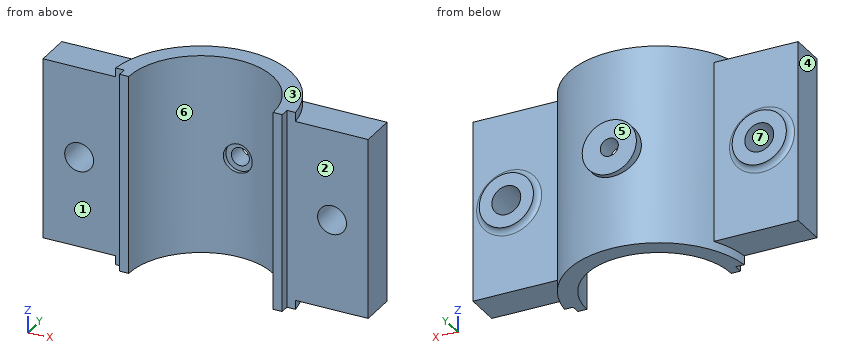
from build123d import *

# Parameters (mm, degrees)
BOSS_EXTRUDE1_DEPTH      = 55
SKETCH2_W                = 180
SKETCH2_H                = 20
BOSS_EXTRUDE2_DEPTH      = 50
SKETCH3_W                = 5
SKETCH3_H                = 5
CUT_EXTRUDE1_DEPTH       = 151.665191733
CUT_EXTRUDE2_DEPTH       = 151.665191733
CUT_EXTRUDE2_DEPTH_BACK  = 151.665191733
SKETCH5_R                = 15
BOSS_EXTRUDE3_DEPTH      = 3
BOSS_EXTRUDE4_REACH      = 120.042
BOSS_EXTRUDE4_END_RADIUS = 50
SKETCH6_R                = 15
HOLE1_D                  = 10
HOLE2_D                  = 16
FILLET1_R                = 3
SKETCH11_R               = 8
CUT_EXTRUDE3_DEPTH       = 42


with BuildPart() as part:
    # Sketch1 → Boss-Extrude1 (new, symmetric)
    with BuildSketch(Plane.XY):
        with BuildLine():
            Line((-50, 0), (50, 0))
            ThreePointArc((50, 0), (0, 50), (-50, 0))
        make_face()
    extrude(amount=BOSS_EXTRUDE1_DEPTH, both=True)

    # Sketch2 → Boss-Extrude2 (add, symmetric)
    with BuildSketch(Plane.XY):
        with Locations((0, 15)):
            Rectangle(SKETCH2_W, SKETCH2_H)
    extrude(amount=BOSS_EXTRUDE2_DEPTH, both=True)

    # Sketch3 → Cut-Extrude1 (cut, symmetric)
    with BuildSketch(Plane.XY.offset(55)):
        with Locations((47.5, 2.5)):
            Rectangle(SKETCH3_W, SKETCH3_H)
    cut_extrude1 = extrude(amount=CUT_EXTRUDE1_DEPTH, both=True, mode=Mode.SUBTRACT)

    # Mirror1: Cut-Extrude1 across plane
    add(cut_extrude1.mirror(Plane(origin=(0, 0, 0), x_dir=(0, 0, 1), z_dir=(1, 0, 0))), mode=Mode.SUBTRACT)

    # Sketch4 → Cut-Extrude2 (cut, two sides: drawn at the far end of the back side and taken through both)
    with BuildSketch(Plane.XY.offset(55).offset(-CUT_EXTRUDE2_DEPTH_BACK)):
        with BuildLine():
            Line((40, 0), (-40, 0))
            ThreePointArc((-40, 0), (0, 40), (40, 0))
        make_face()
    extrude(amount=CUT_EXTRUDE2_DEPTH + CUT_EXTRUDE2_DEPTH_BACK, mode=Mode.SUBTRACT)

    # Sketch5 → Boss-Extrude3 (add)
    with BuildSketch(Plane(origin=(0, 25, 0), x_dir=(1, 0, 0), z_dir=(0, 1, 0))):
        with Locations(Location((-70, 0, 0), (0, 0, 90))):
            Circle(SKETCH5_R)
    boss_extrude3 = extrude(amount=BOSS_EXTRUDE3_DEPTH)

    # Mirror2: Boss-Extrude3 across plane
    add(boss_extrude3.mirror(Plane(origin=(0, 0, 0), x_dir=(0, 0, 1), z_dir=(1, 0, 0))))

    # Boss-Extrude4: up to this cylinder (the profile starts outside it)
    boss_extrude4_end = Plane(origin=(0, 0, 0), z_dir=(0, 0, -1)) * Cylinder(BOSS_EXTRUDE4_END_RADIUS, 341.084, mode=Mode.PRIVATE)
    # Sketch6 → Boss-Extrude4 (add, up to the surface)
    with BuildSketch(Plane(origin=(0, 53, 0), x_dir=(1, 0, 0), z_dir=(0, 1, 0)), mode=Mode.PRIVATE) as boss_extrude4_sk1:
        with Locations(Location((0, 0, 0), (0, 0, 270))):
            Circle(SKETCH6_R)
    boss_extrude4_tool1 = extrude(boss_extrude4_sk1.sketch, amount=-BOSS_EXTRUDE4_REACH, mode=Mode.PRIVATE) - boss_extrude4_end
    add(boss_extrude4_tool1.solids().sort_by_distance((0, 53, 0))[0])

    # Hole1 (through all)
    with Locations(Plane(origin=(0, 53, 0), x_dir=(1, 0, 0), z_dir=(0, 1, 0))):
        with Locations((0, 0)):
            Hole(HOLE1_D / 2)

    # Hole2 (through all)
    with Locations(Plane(origin=(0, 28, 0), x_dir=(1, 0, 0), z_dir=(0, 1, 0))):
        with Locations((-70, 0), (70, 0)):
            Hole(HOLE2_D / 2)

    # Fillet1
    fillet1_edges = [part.edges().sort_by_distance(p)[0] for p in [
        (-70, 25, 15),
        (70, 25, 15),
    ]]
    fillet(fillet1_edges, radius=FILLET1_R - 0.0001)  # a hair under: the kernel refuses the full size

    # Sketch11 → Cut-Extrude3 (cut)
    with BuildSketch(Plane(origin=(0, 0, 0), x_dir=(1, 0, 0), z_dir=(0, 1, 0))):
        with Locations(Location((0, 0, 0), (0, 0, 90))):
            Circle(SKETCH11_R)
    extrude(amount=CUT_EXTRUDE3_DEPTH, mode=Mode.SUBTRACT)


solid = part.part
CAD build for the part. Positions are in the model's coordinates, mm. Face numbers are marked on the shaded views. A direction names the side the tool comes from. Round coordinates to 2 decimals unless told otherwise and drop trailing zeros. Loops run counter-clockwise (first coordinate to the right, second up) from the corner with the lowest first, then second, coordinate; pieces in that order, holes last. Notation, with made-up numbers: M 2.5,-15 L 21.5,-15 A20 cw 21.5,7 Z; hole C -18,48.5 d9. An arc over 180 degrees is marked long. One line per question, with ' | ' between items. Start each with the question number.
Item 1: Pin check, flat tips, straight feed: pin 1 Ø17.5 at (x, z) = (4, 3) entering from -Y; pin 2 Ø1 at (y, z) = (30, 15) entering from +X; pin 3 Ø9 at (x, z) = (77, 7) entering from +Y. Stop position of each tip, or through.
Item 2: Two-plate mould, pull along X, no slides. Class the marked faces 4, 5, 6 and 7: pulls with the +X half, pulls with the -X half, needs draft (parallel to the pull), parting line crosses it, or undercut.
Item 3: Cut at D-D, the plane x = -47.5. Write the cut outline in (y, z), plus the area to 3 significant figures.
Item 4: Cut at C-C, the plane z = -38.5. Write the cut outline in (x, y).
Item 5: Wall check: line 1 (Z direction, x = 0, y = 49); line 2 (Y direction, x = -69, z = 30.5); line 3 (Z direction, x = 56.5, y = 8). Give the ranges that are in metal, low to high.
Item 6: Cut at B-B, the plane y = 20. Write the cut outline in (x, z).
Item 7: Which spindle directions (+Z, -Z, +X, -X, +Y, -Y) get a long thin tool onto all of the face, cutting with end or side? Do the marked faces 1, 2 and 3. Say none if no direction does.
Responses:
1) pin 1: stops at y = 37.91 | pin 2: stops at x = 40.37 | pin 3: stops at y = 28
2) face 4: pulls with the -X half | face 5: needs draft | face 6: undercut | face 7: undercut
3) outline: M 5,-55 L 15.61,-55 L 15.61,-50 L 25,-50 L 25,50 L 15.61,50 L 15.61,55 L 5,55 Z | area: 2,110 mm²
4) outline: M -90,5 L -45,5 L -45,0 L -40,0 A40 cw 40,0 L 45,0 L 45,5 L 90,5 L 90,25 L 43.3,25 A50 ccw -43.3,25 L -90,25 Z
5) line 1: z = -55 to -5, 5 to 55 | line 2: y = 5 to 25 | line 3: z = -50 to 50
6) outline: M -90,-50 L -45.83,-50 L -45.83,-55 L -34.64,-55 L -34.64,55 L -45.83,55 L -45.83,50 L -90,50 Z; M 34.64,-55 L 45.83,-55 L 45.83,-50 L 90,-50 L 90,50 L 45.83,50 L 45.83,55 L 34.64,55 Z; hole C -70,0 d16; hole C 70,0 d16
7) face 1: +Z, -Z, -X, -Y | face 2: +Z, -Z, +X, -Y | face 3: +Z, +X, -X, +Y, -Y
